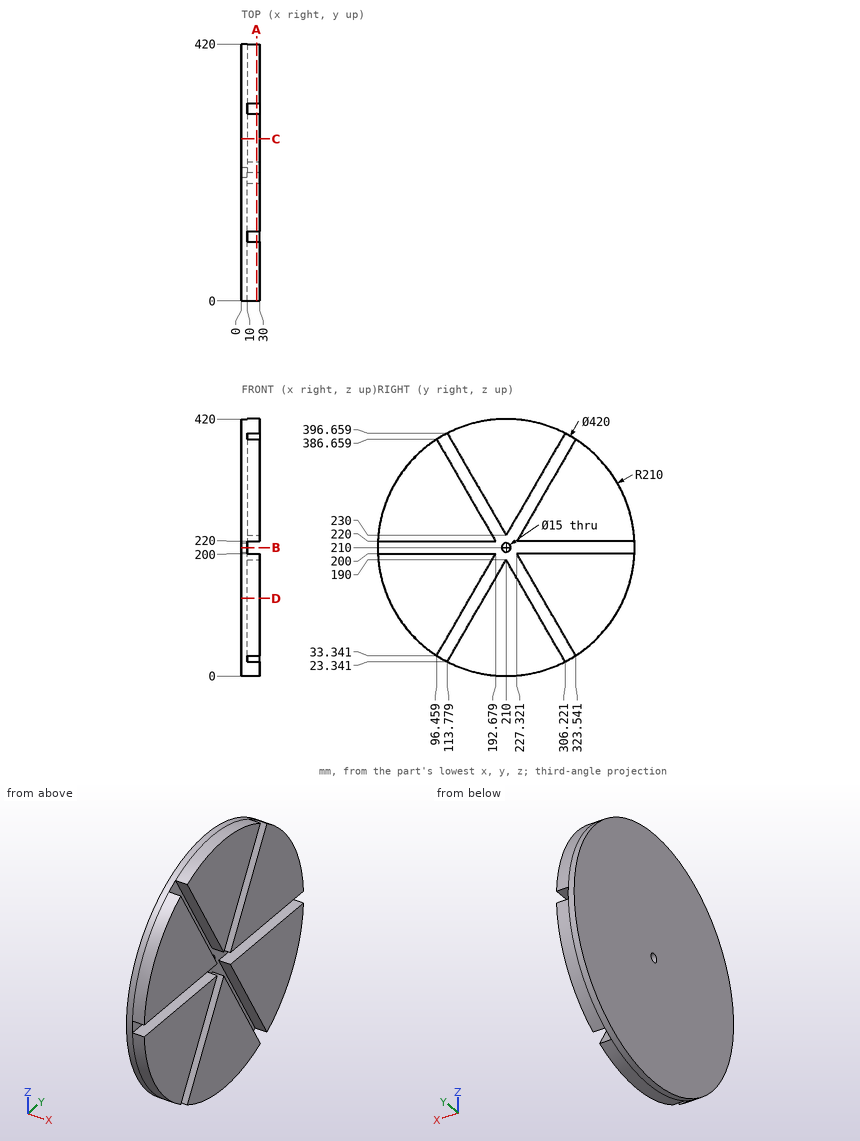
Study the drawing (mm; zero at the part's minimum x, y, z) and answer. Give positions to 0.01 mm unless a question says otherwise; leave off trailing zeros. Write each loop counter-clockwise with the first axis right and the second up, starting at its lowest first coordinate (ties: lowest second). Pieces come first, ordered by that corner, then holes. Notation, with made-up numbers: (26.5, 73) - (68.5, 73) arc R25 ccw to (68.5, 86) - close; hole circle Ø8 at (80, -27). An arc over 180 degrees is marked (long way). Use CSV: the item, a comma, the result in double quotes. Start each with the question number.
(1) Find section B-B (z = 210). Give the vertices of the cut face in (x, y).
(2) Find section A-A (x = 25). Give the vertices of the cut face in (y, z), plus the area to 3 significant figures.
(3) Given P1, Ø1.5, axis at x = 6, z = 259.5, coming from the +Y side; P2, Ø6, axis at x = 20.5, y = 304.5, coming from the -Z side; P3, Ø1.5, axis at x = 23, z = 335, coming from the +Y side, each flat-ended and moving along its own axis, determine where each tip first touches the part or whether it passes through.
(4) Consider line 1 along Z through (x, y) = (6, 210); line 2 along Y through (x, z) = (14, 132) (1 decimal); line 3 along Z through (x, y) = (20, 173.5) (1 decimal). Determine where each line is inside the solid, lowest interval first.
(5) Find section C-C (y = 265). Give the vertices of the cut face in (x, z).
(6) Find section D-D (z = 127). Give the vertices of the cut face in (x, y), plus the area to 4 significant figures.
Findings below:
1,outline,"(0, 0) - (10, 0) - (10, 202.5) - (0, 202.5) - close; (0, 217.5) - (10, 217.5) - (10, 420) - (0, 420) - close"
2,outline,"(0.24, 200) arc R210 ccw to (96.46, 33.34) - (192.68, 200) - close; (0.24, 220) - (192.68, 220) - (96.46, 386.66) arc R210 ccw to start; (113.78, 23.34) arc R210 ccw to (306.22, 23.34) - (210, 190) - close; (113.78, 396.66) - (210, 230) - (306.22, 396.66) arc R210 ccw to start; (227.32, 200) - (323.54, 33.34) arc R210 ccw to (419.76, 200) - close; (227.32, 220) - (419.76, 220) arc R210 ccw to (323.54, 386.66) - close"
2,area,"114,000 mm2"
3,P1,"y = 414.26"
3,P2,"z = 20.98"
3,P3,"y = 379.3"
4,line 1,"0 to 202.5, 217.5 to 420"
4,line 2,"15 to 153.4, 176.5 to 243.5, 266.6 to 405"
4,line 3,"3.2 to 126.8, 166.8 to 200, 220 to 253.2, 293.2 to 416.8"
5,outline,"(0, 7.33) - (30, 7.33) - (30, 94.74) - (10, 94.74) - (10, 134.74) - (30, 134.74) - (30, 200) - (10, 200) - (10, 220) - (30, 220) - (30, 285.26) - (10, 285.26) - (10, 325.26) - (30, 325.26) - (30, 412.67) - (0, 412.67) - close"
6,outline,"(0, 17.1) - (30, 17.1) - (30, 150.53) - (10, 150.53) - (10, 173.63) - (30, 173.63) - (30, 246.37) - (10, 246.37) - (10, 269.47) - (30, 269.47) - (30, 402.9) - (0, 402.9) - close"
6,area,"10,650 mm2"
